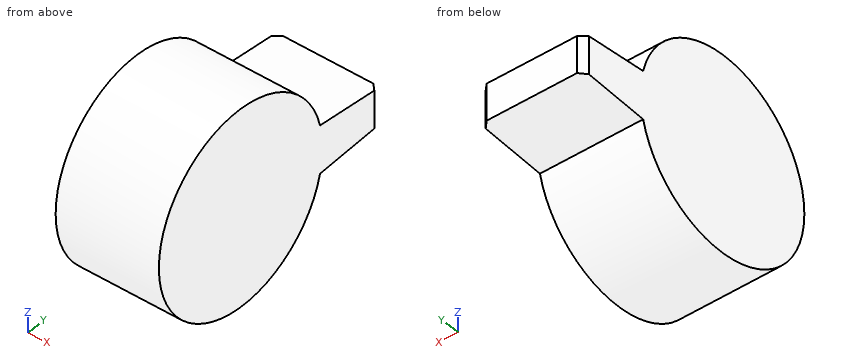
from build123d import *

# Parameters (mm, degrees)
BOSS_EXTRUDE1_DEPTH = 16
CHAMFER1_SIZE       = 1


with BuildPart() as part:
    # Sketch1 → Boss-Extrude1 (new body)
    with BuildSketch(Plane(origin=(0, 0, 0), x_dir=(0, 0, -1), z_dir=(1, 0, 0))):
        with BuildLine():
            Line((-3.65, 14.549140868), (-2.805, 25.5))
            Line((-2.805, 25.5), (2.805, 25.5))
            Line((2.805, 25.5), (3.65, 14.549140868))
            ThreePointArc((3.65, 14.549140868), (0, -15), (-3.65, 14.549140868))
        make_face()
    extrude(amount=BOSS_EXTRUDE1_DEPTH)

    # Chamfer1
    chamfer1_edges = [part.edges().sort_by_distance(p)[0] for p in [
        (0, 25.5, 0),
        (16, 25.5, 0),
    ]]
    chamfer(chamfer1_edges, length=CHAMFER1_SIZE)


solid = part.part
Could you check a few things on this model? Use its own coordinates, in mm. Coordinates: 2 decimals unless noted, no trailing zeros. Loops run counter-clockwise (first coordinate to the right, second up) from the corner with the lowest first, then second, coordinate; pieces in that order, holes last. Notation, with made-up numbers: (37, -29) -> (67, -29) arc R25 cw to (67, -12) -> close; hole circle Ø6 at (74.25, 38). An arc over 180 degrees is marked (long way). Answer in a Markdown table with one row per item.
(1) Imagine slicing it at B-B (y = 20). List the corners of the cut face in (x, z) for me, plus the area to 3 significant figures.
Results found:
| item | result |
|---|---|
| outline | (0, -3.23) -> (16, -3.23) -> (16, 3.23) -> (0, 3.23) -> close |
| area | 103 mm^2 |
(2) If I drill on probe 1 along Y at (x, z) = (3, 12.5); probe 2 along Y at (x, z) = (8, 12.75); probe 3 along Z at (x, y) = (9, 21.5), over which ranges is the centre line in solid material (lowest first)?
Results found:
| item | result |
|---|---|
| probe 1 | y = -8.29 to 8.29 |
| probe 2 | y = -7.9 to 7.9 |
| probe 3 | z = -3.11 to 3.11 |
(3) Will these pins go through, and if not, where does the flat tip stop? pin 1 Ø2 at (x, y) = (2.5, 3) entering from -Z; pin 2 Ø8 at (x, z) = (12.5, -5) entering from -Y.
Results found:
| item | result |
|---|---|
| pin 1 | stops at z = -14.87 |
| pin 2 | stops at y = -14.97 |
(4) Imagine slicing it at A-A (x = 7). List the corners of the cut face in (y, z) for me (3 decimals), plus the area to 3 significant figures.
Results found:
| item | result |
|---|---|
| outline | (14.549, -3.65) -> (25.5, -2.805) -> (25.5, 2.805) -> (14.549, 3.65) arc R15 ccw (long way) to start |
| area | 775 mm^2 |
